```python
from build123d import *

# Parameters (mm, degrees)
BASE_DEPTH         = 2
ESQUISSE2_R        = 1.5
BOSS_FIX_DEPTH     = 2.1
ESQUISSE3_R        = 2
BOSS_BLOCAGE_DEPTH = 1


with BuildPart() as part:
    # Esquisse1 → BASE (new body)
    with BuildSketch(Plane(origin=(0, 0, 0), x_dir=(0, 0, -1), z_dir=(1, 0, 0))):
        with BuildLine():
            Line((2, 25), (2, -25))
            ThreePointArc((2, -25), (0, -27), (-2, -25))
            Line((-2, -25), (-2, 25))
            ThreePointArc((-2, 25), (0, 27), (2, 25))
        make_face()
    extrude(amount=BASE_DEPTH)

    # Esquisse2 → BOSS FIX (add)
    with BuildSketch(Plane(origin=(2, 0, 0), x_dir=(0, 0, -1), z_dir=(1, 0, 0))):
        with Locations(Location((0, 25, 0), (0, 0, 180))):
            Circle(ESQUISSE2_R)
    boss_fix = extrude(amount=BOSS_FIX_DEPTH)

    # Esquisse3 → BOSS BLOCAGE (add)
    with BuildSketch(Plane(origin=(4.1, 0, 0), x_dir=(0, 0, -1), z_dir=(1, 0, 0))):
        with Locations((0, 25)):
            Circle(ESQUISSE3_R)
    boss_blocage = extrude(amount=BOSS_BLOCAGE_DEPTH)

    # SYM FIXATION: BOSS FIX, BOSS BLOCAGE across plane
    add(boss_fix.mirror(Plane.ZX))
    add(boss_blocage.mirror(Plane.ZX))


solid = part.part
```
Geometry: final body of the model. Coordinates: model frame, mm. A direction names the side the tool comes from. Give positions to 0.01 mm unless a question says otherwise; leave off trailing zeros. Write each loop counter-clockwise with the first axis right and the second up, starting at its lowest first coordinate (ties: lowest second). Pieces come first, ordered by that corner, then holes.
1. Reachability of faces 4 (the flat face through (1, 0, -2)), 5 (the cylindrical face through (3.035, -23.513, -0.195)), 6 (the cylindrical face through (4.593, 23.048, 0.434)) from +Z, -Z, +X, -X, +Y, -Y: full face, straight path, thin tool, end or side. Return the list, or none.
2. Section query B-B, the plane z = 0. Return loops of the section in (x, y), then the cut area to 3 significant figures.
3. Line query: probe 1 along Y at (x, z) = (3.35, 0.1); probe 2 along Y at (x, z) = (1.3, -0.2); probe 3 along X at (y, z) = (7, 0.4). Output: solid intervals per line, ascending.
4. Draft query along Y for faces 1 (the flat face through (5.1, 25, 0)), 2 (the cylindrical face through (4.593, -23.048, 0.434)), 3 (the cylindrical face through (1, -27, 0)). Return one class per face: released by +Y, released by -Y, zero draft, split by the parting line, or undercut.
5. Section query A-A, the plane x = 3.1. Return loops of the section in (y, z).
6. Pin query (flat end, axial travel): P1, Ø2, axis at y = 10, z = -0.5, coming from the +X side. Return the tip coordinate at first contact, or that it passes through.
7. Section query C-C, the plane y = 3. Return loops of the section in (x, z).
Computed:
1. face 4: -Z, +X, -X, +Y, -Y
1. face 5: none
1. face 6: +X
2. outline: (0, -27) - (2, -27) - (2, -26.5) - (4.1, -26.5) - (4.1, -27) - (5.1, -27) - (5.1, -23) - (4.1, -23) - (4.1, -23.5) - (2, -23.5) - (2, 23.5) - (4.1, 23.5) - (4.1, 23) - (5.1, 23) - (5.1, 27) - (4.1, 27) - (4.1, 26.5) - (2, 26.5) - (2, 27) - (0, 27) - close
2. area: 129 mm2
3. probe 1: y = -26.5 to -23.5, 23.5 to 26.5
3. probe 2: y = -26.99 to 26.99
3. probe 3: x = 0 to 2
4. face 1: zero draft
4. face 2: undercut
4. face 3: released by -Y
5. outline: circle Ø3 at (-25, 0); circle Ø3 at (25, 0)
6. P1: stops at x = 2
7. outline: (0, -2) - (2, -2) - (2, 2) - (0, 2) - close
